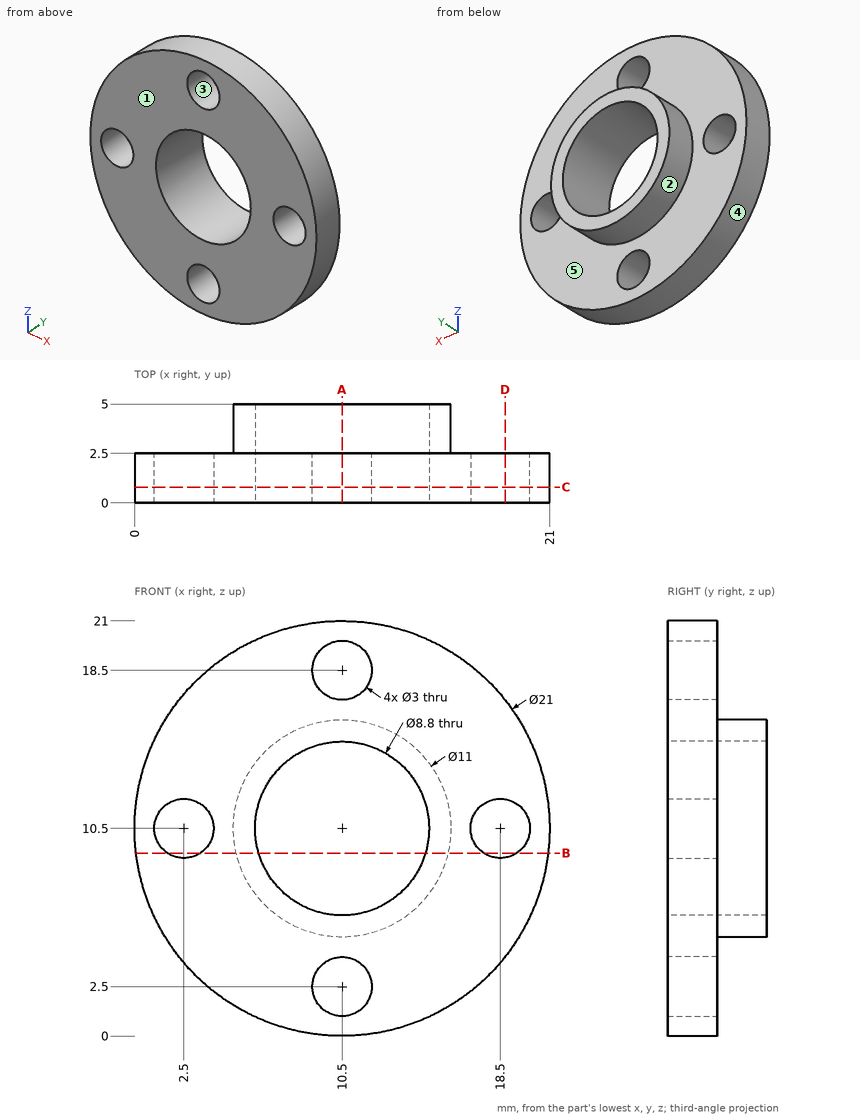
Geometry: see drawing. Coordinates: mm, zero at the bounding-box minimum. A direction names the side the tool comes from. Coordinates: 2 decimals unless noted, no trailing zeros. Loops run counter-clockwise (first coordinate to the right, second up) from the corner with the lowest first, then second, coordinate; pieces in that order, holes last.
(1) First-contact query: pin 1 Ø1 at (y, z) = (0.5, 13.5) entering from +X; pin 2 Ø2 at (y, z) = (2, 19) entering from -X; pin 3 Ø3.5 at (x, z) = (2.5, 10.5) entering from +Y. Flat tips, straight axial feed; report the tip coordinate or a pass-through.
(2) Section A-A on x = 10.5. Return the cut outline in (y, z), then the cut area to 3 significant figures.
(3) Material intervals for probe 1 along Z at (x, y) = (10.5, 2.75); probe 2 along Y at (x, z) = (2.25, 8); probe 3 along X at (y, z) = (3.15, 14), sorted ascending.
(4) Section D-D on x = 18.75. Return the cut outline in (y, z).
(5) Section C-C on y = 0.8. Return the cut outline in (x, z), then the cut area to 3 significant figures.
(6) Pull-direction query (X, two-part tool) for the marked faces 3, 4 and 5; classes: released by +X, released by -X, zero draft, split by the parting line, or undercut.
(7) Section B-B on z = 9.25. Return the cut outline in (x, y), then the cut area to 3 significant figures.
(8) Set-up query: the marked faces 1 and 2. Return all of +Z, -Z, +X, -X, +Y, -Y with unobstructed straight access to the full face (end or side cutting, diameter ignored); none if empty.
Data:
1. pin 1: stops at x = 20.7
1. pin 2: stops at x = 3.15
1. pin 3: stops at y = 2.5
2. outline: (0, 0) - (2.5, 0) - (2.5, 1) - (0, 1) - close; (0, 4) - (2.5, 4) - (2.5, 5) - (5, 5) - (5, 6.1) - (0, 6.1) - close; (0, 14.9) - (5, 14.9) - (5, 16) - (2.5, 16) - (2.5, 17) - (0, 17) - close; (0, 20) - (2.5, 20) - (2.5, 21) - (0, 21) - close
2. area: 21.0 mm2
3. probe 1: z = 5 to 6.1, 14.9 to 16
3. probe 2: y = 0 to 2.5
3. probe 3: x = 6.26 to 7.83, 13.17 to 14.74
4. outline: (0, 4) - (2.5, 4) - (2.5, 9.02) - (0, 9.02) - close; (0, 11.98) - (2.5, 11.98) - (2.5, 17) - (0, 17) - close
5. outline: circle Ø21 at (10.5, 10.5); hole circle Ø3 at (2.5, 10.5); hole circle Ø8.8 at (10.5, 10.5); hole circle Ø3 at (10.5, 2.5); hole circle Ø3 at (10.5, 18.5); hole circle Ø3 at (18.5, 10.5)
5. area: 257 mm2
6. face 3: undercut
6. face 4: split by the parting line
6. face 5: zero draft
7. outline: (0.07, 0) - (1.67, 0) - (1.67, 2.5) - (0.07, 2.5) - close; (3.33, 0) - (6.28, 0) - (6.28, 5) - (5.14, 5) - (5.14, 2.5) - (3.33, 2.5) - close; (14.72, 0) - (17.67, 0) - (17.67, 2.5) - (15.86, 2.5) - (15.86, 5) - (14.72, 5) - close; (19.33, 0) - (20.93, 0) - (20.93, 2.5) - (19.33, 2.5) - close
7. area: 28.4 mm2
8. face 1: +Z, -Z, +X, -X, -Y
8. face 2: +Y
